```python
from build123d import *

# Parameters (mm, degrees)
SKETCH1_W           = 35
SKETCH1_H           = 17
BOSS_EXTRUDE1_DEPTH = 0.5
SKETCH2_W           = 4.5
SKETCH2_H           = 8
BOSS_EXTRUDE2_DEPTH = 3
SKETCH3_W           = 10.6
SKETCH3_H           = 15.6
BOSS_EXTRUDE3_DEPTH = 1.5


with BuildPart() as part:
    # Sketch1 → Boss-Extrude1 (new, symmetric)
    with BuildSketch(Plane(origin=(0, 0, 0), x_dir=(1, 0, 0), z_dir=(0, 1, 0))):
        Rectangle(SKETCH1_W, SKETCH1_H)
    extrude(amount=BOSS_EXTRUDE1_DEPTH, both=True)

    # Sketch2 → Boss-Extrude2 (add)
    with BuildSketch(Plane(origin=(0, 0.5, 0), x_dir=(1, 0, 0), z_dir=(0, 1, 0))):
        with Locations((-15.25, -2.8)):
            Rectangle(SKETCH2_W, SKETCH2_H)
    extrude(amount=BOSS_EXTRUDE2_DEPTH)

    # Sketch3 → Boss-Extrude3 (add)
    with BuildSketch(Plane(origin=(0, 0.5, 0), x_dir=(1, 0, 0), z_dir=(0, 1, 0))):
        with Locations((-0.2, 0.1)):
            Rectangle(SKETCH3_W, SKETCH3_H)
    extrude(amount=BOSS_EXTRUDE3_DEPTH)


solid = part.part
```
The model under review builds one solid part; all positions refer to its coordinate system, in mm. A direction names the side the tool comes from. Round coordinates to 2 decimals unless told otherwise and drop trailing zeros. Order: outer loops, then holes, each group sorted by start corner. A loop starts at its lowest first (then second) coordinate and runs counter-clockwise, first axis right, second up.
(1) Tool access review of faces 5 (the face through (0, 1, 7.7)), 6 (the face through (-15, 2, -1.2)), 7 (the face through (-13, 2, 3)): name each direction out of +Z, -Z, +X, -X, +Y, -Y from which nothing blocks a thin tool from reaching the whole face with its end or side.
Working result:
face 5: +Z, +X, -X, +Y
face 6: -Z, -X, +Y
face 7: +Z, -Z, +Y
(2) Take a section at D-D, the plane z = -0.25. State the section outline as (x, y) points.
Working result:
outline: (-17.5, -0.5) - (17.5, -0.5) - (17.5, 0.5) - (5.1, 0.5) - (5.1, 2) - (-5.5, 2) - (-5.5, 0.5) - (-13, 0.5) - (-13, 3.5) - (-17.5, 3.5) - close
(3) For P1, Ø1.2, axis at y = 1.5, z = 0, coming from the +X side; P2, Ø0.8, axis at x = -2.5, y = 1.5, coming from the +Z side; P3, Ø8, axis at x = 0, z = -4.5, coming from the +Y side; P4, Ø1.6, axis at x = 0.5, y = 1, coming from the -Z side, all flat-tipped, find the tip position at first contact; note any pin that passes through.
Working result:
P1: stops at x = 5.1
P2: stops at z = 7.7
P3: stops at y = 2
P4: stops at z = -8.5
(4) Take a section at C-C, the plane x = 3.5. State the section outline as (y, z) points, plus the area to 3 significant figures.
Working result:
outline: (-0.5, -8.5) - (0.5, -8.5) - (0.5, -7.9) - (2, -7.9) - (2, 7.7) - (0.5, 7.7) - (0.5, 8.5) - (-0.5, 8.5) - close
area: 40.4 mm2
(5) Take a section at A-A, the plane y = 0.85. State the section outline as (x, z) points, plus the area to 3 significant figures.
Working result:
outline: (-17.5, -1.2) - (-13, -1.2) - (-13, 6.8) - (-17.5, 6.8) - close; (-5.5, -7.9) - (5.1, -7.9) - (5.1, 7.7) - (-5.5, 7.7) - close
area: 201 mm2
(6) Mouldability with a two-part tool opening along X and no side actions: class faces 1 (the face through (0, 1, -7.9)), 2 (the face through (-17.5, 1, 2)), 3 (the face through (5.1, 1, 0)), 4 (the face through (8, 0.5, 0)) as released by +X, released by -X, zero draft, split by the parting line, or undercut.
Working result:
face 1: zero draft
face 2: released by -X
face 3: released by +X
face 4: undercut
(7) Take a section at B-B, the plane z = -3. State the section outline as (x, y) points.
Working result:
outline: (-17.5, -0.5) - (17.5, -0.5) - (17.5, 0.5) - (5.1, 0.5) - (5.1, 2) - (-5.5, 2) - (-5.5, 0.5) - (-17.5, 0.5) - close
(8) Wall thickness on L1, parallel to X at y = 1.9, z = 1.5; L2, parallel to X at y = 2.15, z = 0.75; L3, parallel to Y at x = -13, z = -5: over which ranges is each line inside the solid? List them lowest first.
Working result:
L1: x = -17.5 to -13, -5.5 to 5.1
L2: x = -17.5 to -13
L3: y = -0.5 to 0.5
